Here's how the part is built. I have some questions about the finished solid (model axes, mm). Coordinates: 2 decimals unless noted, no trailing zeros. Loops run counter-clockwise (first coordinate to the right, second up) from the corner with the lowest first, then second, coordinate; pieces in that order, holes last. Notation, with made-up numbers: (10, -38) - (36, -38) arc R27 ccw to (36, -14) - close; hole circle Ø8 at (-7.5, 54). An arc over 180 degrees is marked (long way). Use a Markdown table: item, result.
```python
from build123d import *

# Parameters (mm, degrees)
BOSS_EXTRUDE1_OUTLINE_R   = 100
BOSS_EXTRUDE1_OUTLINE_R_2 = 2.1
BOSS_EXTRUDE1_OUTLINE_W   = 26
BOSS_EXTRUDE1_OUTLINE_H   = 34
BOSS_EXTRUDE1_DEPTH       = 6.35
SKETCH2_R                 = 2.1
CUT_EXTRUDE1_DEPTH        = 6.35
CUT_EXTRUDE4_DEPTH        = 6.35
BOSS_EXTRUDE2_DEPTH       = 6.35
SKETCH4_R                 = 1.35
CUT_EXTRUDE3_DEPTH        = 6.35
SKETCH7_R                 = 2.1
BOSS_EXTRUDE3_DEPTH       = 6.35
SKETCH8_R                 = 2.1
CUT_EXTRUDE5_DEPTH        = 6.35


# Read off the part's stored shape, not the designer's step: Boss-Extrude1
with BuildPart() as part:
    # Boss-Extrude1 outline → Boss-Extrude1 (new body)
    with BuildSketch(Plane(origin=(0, 0, 0), x_dir=(1, 0, 0), z_dir=(0, 1, 0))):
        Circle(BOSS_EXTRUDE1_OUTLINE_R)
        with Locations((-69.915362552, -64.90303983)):
            Circle(BOSS_EXTRUDE1_OUTLINE_R_2, mode=Mode.SUBTRACT)
        with Locations((-59.523057707, -58.90303983)):
            Circle(BOSS_EXTRUDE1_OUTLINE_R_2, mode=Mode.SUBTRACT)
        with Locations((-91.165362552, -28.09696017)):
            Circle(BOSS_EXTRUDE1_OUTLINE_R_2, mode=Mode.SUBTRACT)
        with Locations((-80.773057707, -22.09696017)):
            Circle(BOSS_EXTRUDE1_OUTLINE_R_2, mode=Mode.SUBTRACT)
        Polygon((-56.719854476, -47.758330249), (-69.719854476, -25.241669751), (-40.274990748, -8.241669751), (-27.274990748, -30.758330249), align=None, mode=Mode.SUBTRACT)
        with Locations((69.915362552, -64.90303983)):
            Circle(BOSS_EXTRUDE1_OUTLINE_R_2, mode=Mode.SUBTRACT)
        with Locations((59.523057707, -58.90303983)):
            Circle(BOSS_EXTRUDE1_OUTLINE_R_2, mode=Mode.SUBTRACT)
        Polygon((69.719854476, -25.241669751), (56.719854476, -47.758330249), (27.274990748, -30.758330249), (40.274990748, -8.241669751), align=None, mode=Mode.SUBTRACT)
        with Locations((91.165362552, -28.09696017)):
            Circle(BOSS_EXTRUDE1_OUTLINE_R_2, mode=Mode.SUBTRACT)
        with Locations((80.773057707, -22.09696017)):
            Circle(BOSS_EXTRUDE1_OUTLINE_R_2, mode=Mode.SUBTRACT)
        with Locations((-21.25, 81)):
            Circle(BOSS_EXTRUDE1_OUTLINE_R_2, mode=Mode.SUBTRACT)
        with Locations((-21.25, 93)):
            Circle(BOSS_EXTRUDE1_OUTLINE_R_2, mode=Mode.SUBTRACT)
        with Locations((0, 56)):
            Rectangle(BOSS_EXTRUDE1_OUTLINE_W, BOSS_EXTRUDE1_OUTLINE_H, mode=Mode.SUBTRACT)
        with Locations((21.25, 81)):
            Circle(BOSS_EXTRUDE1_OUTLINE_R_2, mode=Mode.SUBTRACT)
        with Locations((21.25, 93)):
            Circle(BOSS_EXTRUDE1_OUTLINE_R_2, mode=Mode.SUBTRACT)
    extrude(amount=BOSS_EXTRUDE1_DEPTH)

    # Sketch2 → Cut-Extrude1 (cut)
    with BuildSketch(Plane(origin=(0, 6.35, 0), x_dir=(1, 0, 0), z_dir=(0, 1, 0))):
        with Locations(Location((0, -94, 0), (0, 0, 270))):
            Circle(SKETCH2_R)
        with Locations(Location((-81.406387956, 47, 0), (0, 0, 270))):
            Circle(SKETCH2_R)
        with Locations(Location((81.406387956, 47, 0), (0, 0, 270))):
            Circle(SKETCH2_R)
    extrude(amount=-CUT_EXTRUDE1_DEPTH, mode=Mode.SUBTRACT)

    # Sketch5 → Cut-Extrude4 (cut)
    with BuildSketch(Plane(origin=(0, 6.35, 0), x_dir=(1, 0, 0), z_dir=(0, 1, 0))):
        with BuildLine():
            Line((26.502570178, 77.23282604), (21.101148971, 15.494299138))
            ThreePointArc((21.101148971, 15.494299138), (21.751995443, 12.558520424), (23.969031153, 10.526981489))
            Line((23.969031153, 10.526981489), (80.136874446, -15.664513981))
            ThreePointArc((80.136874446, -15.664513981), (84.646931723, -15.520976202), (87.204782969, -11.803636193))
            ThreePointArc((87.204782969, -11.803636193), (76.210235533, 44), (33.380142684, 81.423375479))
            ThreePointArc((33.380142684, 81.423375479), (28.881906179, 81.066881325), (26.502570178, 77.23282604))
        make_face()
        with BuildLine():
            Line((53.634304268, -61.56831206), (2.867882182, -26.021280627))
            ThreePointArc((2.867882182, -26.021280627), (0, -25.117040848), (-2.867882182, -26.021280627))
            Line((-2.867882182, -26.021280627), (-53.634304268, -61.56831206))
            ThreePointArc((-53.634304268, -61.56831206), (-55.765025544, -65.545905124), (-53.824640284, -69.619739286))
            ThreePointArc((-53.824640284, -69.619739286), (0, -88), (53.824640284, -69.619739286))
            ThreePointArc((53.824640284, -69.619739286), (55.765025544, -65.545905124), (53.634304268, -61.56831206))
        make_face()
        with BuildLine():
            Line((-80.136874446, -15.664513981), (-23.969031153, 10.526981489))
            ThreePointArc((-23.969031153, 10.526981489), (-21.751995443, 12.558520424), (-21.101148971, 15.494299138))
            Line((-21.101148971, 15.494299138), (-26.502570178, 77.23282604))
            ThreePointArc((-26.502570178, 77.23282604), (-28.881906179, 81.066881325), (-33.380142684, 81.423375479))
            ThreePointArc((-33.380142684, 81.423375479), (-76.210235533, 44), (-87.204782969, -11.803636193))
            ThreePointArc((-87.204782969, -11.803636193), (-84.646931723, -15.520976202), (-80.136874446, -15.664513981))
        make_face()
    extrude(amount=-CUT_EXTRUDE4_DEPTH, mode=Mode.SUBTRACT)

    # Sketch6 → Boss-Extrude2 (add)
    with BuildSketch(Plane(origin=(0, 6.35, 0), x_dir=(1, 0, 0), z_dir=(0, 1, 0))):
        with BuildLine():
            Line((-24.5, 38.25), (-23.092014827, 38.25))
            Line((-23.092014827, 38.25), (-22.392105519, 30.25))
            Line((-22.392105519, 30.25), (-24.5, 30.25))
            ThreePointArc((-24.5, 30.25), (-28.5, 34.25), (-24.5, 38.25))
        make_face()
        with BuildLine():
            Line((22.392105519, 30.25), (24.5, 30.25))
            ThreePointArc((24.5, 30.25), (28.5, 34.25), (24.5, 38.25))
            Line((24.5, 38.25), (23.092014827, 38.25))
            Line((23.092014827, 38.25), (22.392105519, 30.25))
        make_face()
    extrude(amount=-BOSS_EXTRUDE2_DEPTH)

    # Sketch4 → Cut-Extrude3 (cut)
    with BuildSketch(Plane(origin=(0, 6.35, 0), x_dir=(1, 0, 0), z_dir=(0, 1, 0))):
        with Locations(Location((-24.5, -23.75, 0), (0, 0, 270))):
            Circle(SKETCH4_R)
        with Locations(Location((24.5, -23.75, 0), (0, 0, 270))):
            Circle(SKETCH4_R)
        with Locations(Location((24.5, 34.25, 0), (0, 0, 270))):
            Circle(SKETCH4_R)
        with Locations(Location((-24.5, 34.25, 0), (0, 0, 270))):
            Circle(SKETCH4_R)
    extrude(amount=-CUT_EXTRUDE3_DEPTH, mode=Mode.SUBTRACT)

    # Sketch7 → Boss-Extrude3 (add)
    # profile 1 of 2: a face of its own
    with BuildSketch(Plane(origin=(0, 6.35, 0), x_dir=(1, 0, 0), z_dir=(0, 1, 0))):
        with BuildLine():
            Line((67.127718677, 2), (17.894755671, 2))
            Line((17.894755671, 2), (17.894755671, -2))
            Line((17.894755671, -2), (67.127718677, -2))
            ThreePointArc((67.127718677, -2), (70, -3.5), (72.872281323, -2))
            Line((72.872281323, -2), (93.633289792, -2))
            Line((93.633289792, -2), (93.633289792, 2))
            Line((93.633289792, 2), (72.872281323, 2))
            ThreePointArc((72.872281323, 2), (70, 3.5), (67.127718677, 2))
        make_face()
        with Locations(Location((70, 0, 0), (0, 0, 270))):
            Circle(SKETCH7_R, mode=Mode.SUBTRACT)
    # profile 2 of 2: a face of its own
    with BuildSketch(Plane(origin=(0, 6.35, 0), x_dir=(1, 0, 0), z_dir=(0, 1, 0))):
        with BuildLine():
            Line((-72.872281323, -2), (-93.633289792, -2))
            Line((-93.633289792, -2), (-93.633289792, 2))
            Line((-93.633289792, 2), (-72.872281323, 2))
            ThreePointArc((-72.872281323, 2), (-70, 3.5), (-67.127718677, 2))
            Line((-67.127718677, 2), (-17.894755671, 2))
            Line((-17.894755671, 2), (-17.894755671, -2))
            Line((-17.894755671, -2), (-67.127718677, -2))
            ThreePointArc((-67.127718677, -2), (-70, -3.5), (-72.872281323, -2))
        make_face()
        with Locations(Location((-70, 0, 0), (0, 0, 270))):
            Circle(SKETCH7_R, mode=Mode.SUBTRACT)
    extrude(amount=-BOSS_EXTRUDE3_DEPTH)

    # Sketch8 → Cut-Extrude5 (cut)
    with BuildSketch(Plane(origin=(0, 6.35, 0), x_dir=(1, 0, 0), z_dir=(0, 1, 0))):
        with Locations(Location((27, 0, 0), (0, 0, 270))):
            Circle(SKETCH8_R)
        with Locations(Location((-27, 0, 0), (0, 0, 270))):
            Circle(SKETCH8_R)
    extrude(amount=-CUT_EXTRUDE5_DEPTH, mode=Mode.SUBTRACT)


solid = part.part
```
Q1. Will these pins go through, and if not, where does the flat tip stop? P1, Ø2.5, axis at x = -91.17, z = 28.1, coming from the +Y side; P2, Ø1.9, axis at x = -83, y = 2, coming from the +Z side; P3, Ø1.5, axis at x = 47.5, y = 5.5, coming from the -Z side.
Check values:
| item | result |
|---|---|
| P1 | through |
| P2 | z = 57.16 |
| P3 | z = -88.4 |
Q2. Please list where these lines run through material, in increasing order: L1, parallel to X at y = 2.25, z = 0; L2, parallel to Z at x = -9, y = 6; L3, parallel to X at y = 5.25, z = -7. Write a range as from..to.
Check values:
| item | result |
|---|---|
| L1 | -100..-72.1, -67.9..-29.1, -24.9..24.9, 29.1..67.9, 72.1..100 |
| L2 | -99.59..-73, -39..30.32, 87.54..99.59 |
| L3 | -99.75..-87.72, -31.53..31.53, 87.72..99.75 |
Q3. If we mould it in two halves opening along Z, with no side actions, what happens to faces 1 (the face through (13, 3, -56)), 2 (the face through (95.38, 3.13, -30.04))? For each: pulls with the +Z half, pulls with the -Z half, needs draft (parallel to the pull), parting line crosses it, or undercut.
Check values:
| item | result |
|---|---|
| face 1 | undercut |
| face 2 | parting line crosses it |
Q4. I want a section at B-B, the plane z = -18. Write out the boundary of the cut face in (x, y).
Check values:
| item | result |
|---|---|
| outline | (-98.37, 0) - (-86.14, 0) - (-86.14, 6.35) - (-98.37, 6.35) - close; (-21.32, 0) - (21.32, 0) - (21.32, 6.35) - (-21.32, 6.35) - close; (86.14, 0) - (98.37, 0) - (98.37, 6.35) - (86.14, 6.35) - close |
Q5. I want a section at A-A, the plane x = -64. Write out the boundary of the cut face in (y, z).
Check values:
| item | result |
|---|---|
| outline | (0, -76.84) - (6.35, -76.84) - (6.35, -60.4) - (0, -60.4) - close; (0, -2) - (6.35, -2) - (6.35, 2) - (0, 2) - close; (0, 8.14) - (6.35, 8.14) - (6.35, 21.94) - (0, 21.94) - close; (0, 35.15) - (6.35, 35.15) - (6.35, 76.84) - (0, 76.84) - close |
Q6. I want a section at C-C, the plane z = 72. Write out the boundary of the cut face in (x, y), then the cut area to 3 significant figures.
Check values:
| item | result |
|---|---|
| outline | (-69.4, 0) - (-50.6, 0) - (-50.6, 6.35) - (-69.4, 6.35) - close; (50.6, 0) - (69.4, 0) - (69.4, 6.35) - (50.6, 6.35) - close |
| area | 239 mm^2 |
Q7. I want a section at D-D, the plane y = 1.5. Give the number of separate pieces and of enclosed holes in the cut face, then the cut area to 3 significant figures.
Check values:
| item | result |
|---|---|
| separate pieces | 1 |
| enclosed holes | 31 |
| area | 16,200 mm^2 |
